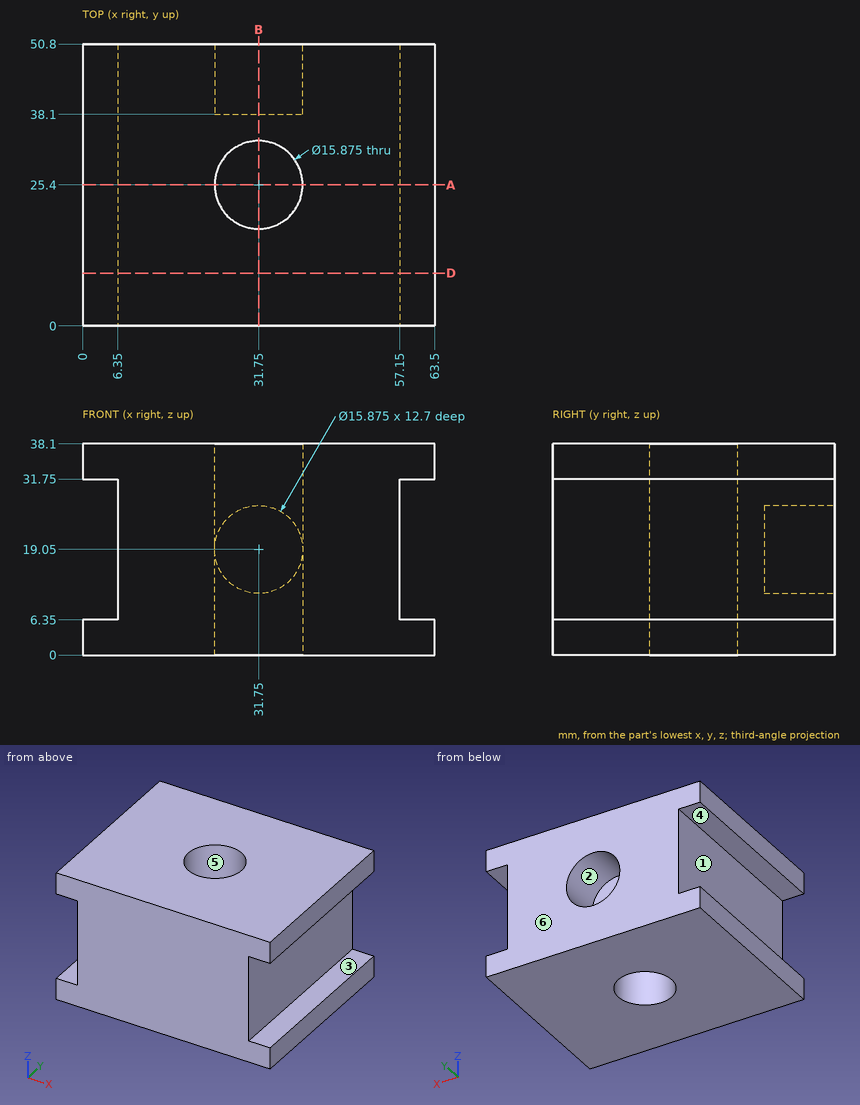
Input: dimensioned drawing with shaded views. Units: mm. Origin: part minimum x, y, z. A direction names the side the tool comes from. Coordinates: 2 decimals unless noted, no trailing zeros. Write each loop counter-clockwise with the first axis right and the second up, starting at its lowest first coordinate (ties: lowest second). Pieces come first, ordered by that corner, then holes. Notation, with made-up numbers: M -23.5,-29 L -19.5,-29 A22 ccw -19.5,-11 Z; hole C 21,51.25 d7. An arc over 180 degrees is marked long. Use one line per item in the form item = value.
Q1. Set-up query: the marked faces 1, 2 and 3. Return all of +Z, -Z, +X, -X, +Y, -Y with unobstructed straight access to the full face (end or side cutting, diameter ignored); none if empty.
Answer below:
face_1 = -X, +Y, -Y
face_2 = +Y
face_3 = +X, +Y, -Y
Q2. Section B-B (x = 31.75). Return loops of the section in (y, z), plus the area to 3 significant figures.
Answer below:
outline = M 0,0 L 17.46,0 L 17.46,38.1 L 0,38.1 Z; M 33.34,0 L 50.8,0 L 50.8,11.11 L 38.1,11.11 L 38.1,26.99 L 50.8,26.99 L 50.8,38.1 L 33.34,38.1 Z
area = 1,130 mm²
Q3. Draft query along Y for the marked faces 4, 5 and 6. Return one class per face: released by +Y, released by -Y, zero draft, split by the parting line, or undercut.
Answer below:
face_4 = zero draft
face_5 = undercut
face_6 = released by +Y
Q4. First-contact query: pin 1 (8 mm diameter, centred on y = 25, z = 10.5, fed in from +X); pin 2 (5 mm diameter, centred on y = 29.5, z = 24, fed in from -X); pin 3 (9.5 mm diameter, centred on x = 31.75, z = 19.05, fed in from +Y). Flat tips, straight axial feed; report the tip coordinate or a pass-through.
Answer below:
pin_1 = 57.15
pin_2 = 6.35
pin_3 = 38.1
Q5. Section D-D (y = 9.5). Return loops of the section in (x, z), plus the area to 3 significant figures.
Answer below:
outline = M 0,0 L 63.5,0 L 63.5,6.35 L 57.15,6.35 L 57.15,31.75 L 63.5,31.75 L 63.5,38.1 L 0,38.1 L 0,31.75 L 6.35,31.75 L 6.35,6.35 L 0,6.35 Z
area = 2,100 mm²
Q6. Material intervals for probe 1 along X at (y, z) = (25, 22); probe 2 along Z at (x, y) = (31.75, 47); probe 3 along X at (y, z) = (39.5, 31.5), sorted ascending. Write a range as from..to.
Answer below:
probe_1 = 6.35..23.82, 39.68..57.15
probe_2 = 0..11.11, 26.99..38.1
probe_3 = 6.35..57.15
Q7. Section A-A (y = 25.4). Return loops of the section in (x, z), plus the area to 3 significant figures.
Answer below:
outline = M 0,0 L 23.81,0 L 23.81,38.1 L 0,38.1 L 0,31.75 L 6.35,31.75 L 6.35,6.35 L 0,6.35 Z; M 39.69,0 L 63.5,0 L 63.5,6.35 L 57.15,6.35 L 57.15,31.75 L 63.5,31.75 L 63.5,38.1 L 39.69,38.1 Z
area = 1,490 mm²
